```python
from build123d import *

# Parameters (mm, degrees)
F0_R     = 138.5
F1_DEPTH = 20
F2_R     = 40
F3_DEPTH = 25
F5_DEPTH = 25
F7_DEPTH = 20.001


with BuildPart() as f1:
    # F0 (on Top) → F1 (new body)
    with BuildSketch(Plane.XY):
        Circle(F0_R)
    extrude(amount=F1_DEPTH)

    # F2 (on face) → F3 (cut)
    with BuildSketch(Plane.XY.offset(20)):
        Circle(F2_R)
    extrude(amount=-F3_DEPTH, mode=Mode.SUBTRACT)

    # F4 (on face) → F5 (cut)
    with BuildSketch(Plane.XY.offset(20)):
        with BuildLine():
            ThreePointArc((-2.4994574064, 59.9479166667), (0, 60), (2.4994574064, 59.9479166667))
            ThreePointArc((2.4994574064, 59.9479166667), (2.4998643479, 59.9739569202), (2.5, 60))
            ThreePointArc((2.5, 60), (-0.0260430798, 62.4998643479), (-2.4994574064, 59.9479166667))
        make_face()
        with BuildLine():
            ThreePointArc((-2.4994574064, 59.9479166667), (0, 57.5), (2.4994574064, 59.9479166667))
            ThreePointArc((2.4994574064, 59.9479166667), (0, 60), (-2.4994574064, 59.9479166667))
        make_face()
        with BuildLine():
            ThreePointArc((-57.5, 0), (-58.2139137292, 1.7492557941), (-59.9479166667, 2.4994574064))
            ThreePointArc((-59.9479166667, 2.4994574064), (-60, 0), (-59.9479166667, -2.4994574064))
            ThreePointArc((-59.9479166667, -2.4994574064), (-58.2139137292, -1.7492557941), (-57.5, 0))
        make_face()
        with BuildLine():
            ThreePointArc((-59.9479166667, -2.4994574064), (-60, 0), (-59.9479166667, 2.4994574064))
            ThreePointArc((-59.9479166667, 2.4994574064), (-62.5, 0), (-59.9479166667, -2.4994574064))
        make_face()
        with BuildLine():
            ThreePointArc((59.9479166667, 2.4994574064), (59.9869777535, 1.25), (60, 0))
            ThreePointArc((60, 0), (59.9869777535, -1.25), (59.9479166667, -2.4994574064))
            ThreePointArc((59.9479166667, -2.4994574064), (61.7492557941, -1.7860862708), (62.5, 0))
            ThreePointArc((62.5, 0), (61.7492557941, 1.7860862708), (59.9479166667, 2.4994574064))
        make_face()
        with BuildLine():
            ThreePointArc((59.9479166667, -2.4994574064), (59.9869777535, -1.25), (60, 0))
            ThreePointArc((60, 0), (59.9869777535, 1.25), (59.9479166667, 2.4994574064))
            ThreePointArc((59.9479166667, 2.4994574064), (57.5, 0), (59.9479166667, -2.4994574064))
        make_face()
        with BuildLine():
            ThreePointArc((2.5, -60), (2.4998643479, -59.9739569202), (2.4994574064, -59.9479166667))
            ThreePointArc((2.4994574064, -59.9479166667), (0, -60), (-2.4994574064, -59.9479166667))
            ThreePointArc((-2.4994574064, -59.9479166667), (-0.0260430798, -62.4998643479), (2.5, -60))
        make_face()
        with BuildLine():
            ThreePointArc((-2.4994574064, -59.9479166667), (0, -60), (2.4994574064, -59.9479166667))
            ThreePointArc((2.4994574064, -59.9479166667), (0, -57.5), (-2.4994574064, -59.9479166667))
        make_face()
    extrude(amount=-F5_DEPTH, mode=Mode.SUBTRACT)

    # F6 (on face) → F7 (cut, through all)
    with BuildSketch(Plane.XY.offset(20)):
        with BuildLine():
            ThreePointArc((-2.499860907, 118.473628692), (0, 118.5), (2.499860907, 118.473628692))
            ThreePointArc((2.499860907, 118.473628692), (2.4999652265, 118.4868141626), (2.5, 118.5))
            ThreePointArc((2.5, 118.5), (-0.0131858374, 120.9999652265), (-2.499860907, 118.473628692))
        make_face()
        with BuildLine():
            ThreePointArc((-2.499860907, 118.473628692), (0, 116), (2.499860907, 118.473628692))
            ThreePointArc((2.499860907, 118.473628692), (0, 118.5), (-2.499860907, 118.473628692))
        make_face()
        with BuildLine():
            ThreePointArc((-116, 0), (-116.7229338406, 1.7584185693), (-118.473628692, 2.499860907))
            ThreePointArc((-118.473628692, 2.499860907), (-118.5, 0), (-118.473628692, -2.499860907))
            ThreePointArc((-118.473628692, -2.499860907), (-116.7229338406, -1.7584185693), (-116, 0))
        make_face()
        with BuildLine():
            ThreePointArc((-118.473628692, -2.499860907), (-118.5, 0), (-118.473628692, 2.499860907))
            ThreePointArc((-118.473628692, 2.499860907), (-121, 0), (-118.473628692, -2.499860907))
        make_face()
        with BuildLine():
            ThreePointArc((-2.499860907, -118.473628692), (0, -118.5), (2.499860907, -118.473628692))
            ThreePointArc((2.499860907, -118.473628692), (0, -116), (-2.499860907, -118.473628692))
        make_face()
        with BuildLine():
            ThreePointArc((2.5, -118.5), (2.4999652265, -118.4868141626), (2.499860907, -118.473628692))
            ThreePointArc((2.499860907, -118.473628692), (0, -118.5), (-2.499860907, -118.473628692))
            ThreePointArc((-2.499860907, -118.473628692), (-0.0131858374, -120.9999652265), (2.5, -118.5))
        make_face()
        with BuildLine():
            ThreePointArc((118.473628692, -2.499860907), (118.4934069896, -1.25), (118.5, 0))
            ThreePointArc((118.5, 0), (118.4934069896, 1.25), (118.473628692, 2.499860907))
            ThreePointArc((118.473628692, 2.499860907), (116, 0), (118.473628692, -2.499860907))
        make_face()
        with BuildLine():
            ThreePointArc((118.473628692, 2.499860907), (118.4934069896, 1.25), (118.5, 0))
            ThreePointArc((118.5, 0), (118.4934069896, -1.25), (118.473628692, -2.499860907))
            ThreePointArc((118.473628692, -2.499860907), (120.2584185693, -1.7770661594), (121, 0))
            ThreePointArc((121, 0), (120.2584185693, 1.7770661594), (118.473628692, 2.499860907))
        make_face()
    extrude(amount=-F7_DEPTH, mode=Mode.SUBTRACT)


solid = f1.part
```
Input: part model. Units: mm. Frame: model coordinates. Give positions to 0.01 mm unless a question says otherwise; leave off trailing zeros. Order: outer loops, then holes, each group sorted by start corner. A loop starts at its lowest first (then second) coordinate and runs counter-clockwise, first axis right, second up.
1. Material intervals for L1, parallel to Y at x = 116.5, z = 6; L2, parallel to Y at x = 31.5, z = 14.75; L3, parallel to X at y = -9, z = 3, sorted ascending.
Derived:
L1: y = -74.9 to -1.5, 1.5 to 74.9
L2: y = -134.87 to -24.65, 24.65 to 134.87
L3: x = -138.21 to -38.97, 38.97 to 138.21
2. Section D-D on x = 103. Return the cut outline in (y, z).
Derived:
outline: (-92.59, 0) - (92.59, 0) - (92.59, 20) - (-92.59, 20) - close
3. Section B-B on x = -6.5. Return the cut outline in (y, z), and give its area (3 significant figures).
Derived:
outline: (-138.35, 0) - (-39.47, 0) - (-39.47, 20) - (-138.35, 20) - close; (39.47, 0) - (138.35, 0) - (138.35, 20) - (39.47, 20) - close
area: 3,960 mm2
4. Section A-A on z = 5.75. Give the number of separate pieces and of enclosed holes in the cut face, and give its area (3 significant figures).
Derived:
separate pieces: 1
enclosed holes: 9
area: 55,100 mm2
5. Pin query (flat end, axial travel): pin 1 (1 mm diameter, centred on x = 72, z = 9, fed in from +Y); pin 2 (8 mm diameter, centred on y = -11.5, z = 14, fed in from -X); pin 3 (1 mm diameter, centred on x = 101.5, z = 13, fed in from +Y); pin 4 (10 mm diameter, centred on x = -36.5, y = -22, fed in from -Z). Return the tip coordinate at first contact, or that it passes through.
Derived:
pin 1: stops at y = 118.62
pin 2: stops at x = -138.3
pin 3: stops at y = 94.77
pin 4: stops at z = 0
6. Section C-C on y = -92. Return the cut outline in (x, z).
Derived:
outline: (-103.53, 0) - (103.53, 0) - (103.53, 20) - (-103.53, 20) - close
7. Mould query, pull axis Y, two halves, no side actions, for faces 1 (the cylindrical face through (-8.67, -39.05, 10.14)), 2 (the cylindrical face through (-18.03, 137.32, 9.86)), 3 (the flat face through (29, -29, 20)). Classes: released by +Y, released by -Y, zero draft, split by the parting line, or undercut.
Derived:
face 1: undercut
face 2: split by the parting line
face 3: zero draft
